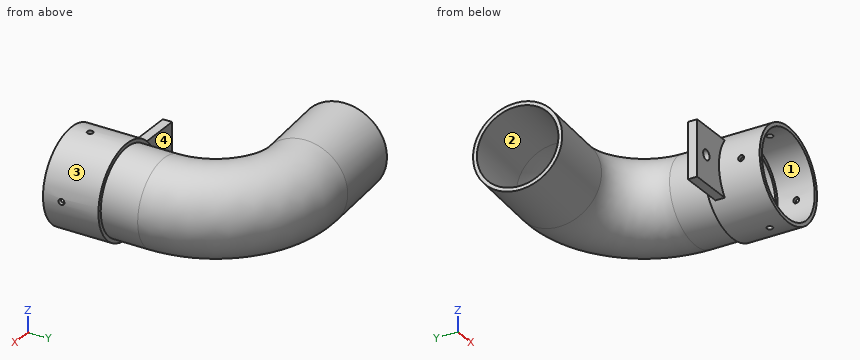
```python
from build123d import *

# Parameters (mm, degrees)
SKETCH_1_R               = 23
SKETCH_1_R_2             = 21
EXTRUDE_1_DEPTH          = 20
EXTRUDE_1_DEPTH_BACK     = 10
SKETCH_3_R               = 25
SKETCH_3_R_2             = 23
SKETCH_5_R               = 2.75
EXTRUDE_3_DEPTH          = 5
CUT_EXTRUDE_1_DEPTH      = 136.900654152
CUT_EXTRUDE_1_DEPTH_BACK = 136.900654152
SKETCH_6_R               = 1.6
CUT_EXTRUDE_2_DEPTH      = 136.900654171
CUT_EXTRUDE_2_DEPTH_BACK = 136.900654171
SKETCH_7_R               = 1.6


with BuildPart() as part:
    # Sweep 1: sweep along a path in Sketch 2
    with BuildLine(Plane.XY) as sweep_1_path:
        Line((0, 0), (0, 30))
        ThreePointArc((0, 30), (-14.598440657, 63.177480156), (-48.922008424, 74.828761414))
        Line((-48.922008424, 74.828761414), (-88.769796347, 71.342531704))
    # Sketch 1 → Sweep 1 (sweep)
    with BuildSketch(Plane(origin=(0, 0, 0), x_dir=(1, 0, 0), z_dir=(0, 1, 0))):
        Circle(SKETCH_1_R)
        Circle(SKETCH_1_R_2, mode=Mode.SUBTRACT)
    sweep(path=sweep_1_path.line)


with BuildPart() as body_2:
    # Sketch 3 → Extrude 1 (new, two sides: drawn at the far end of the back side and taken through both)
    with BuildSketch(Plane(origin=(0, 0, 58.765701135), x_dir=(1, 0, 0), z_dir=(0, -1, 0)).offset(-EXTRUDE_1_DEPTH_BACK)):
        with Locations(Location((0, -58.765701135, 0), (0, 0, 270))):
            Circle(SKETCH_3_R)
        with Locations(Location((0, -58.765701135, 0), (0, 0, 270))):
            Circle(SKETCH_3_R_2, mode=Mode.SUBTRACT)
    extrude(amount=EXTRUDE_1_DEPTH + EXTRUDE_1_DEPTH_BACK)


    add(part.part)  # Extrude 3 merges part
    # Sketch 5 → Extrude 3 (add)
    with BuildSketch(Plane(origin=(0, 2, 0), x_dir=(-1, 0, 0), z_dir=(0, -1, 0))):
        with BuildLine():
            Line((20, 15), (44, 15))
            Line((44, 15), (44, -15))
            Line((44, -15), (20, -15))
            ThreePointArc((20, -15), (25, 0), (20, 15))
        make_face()
        with Locations(Location((36, 0, 0), (0, 0, 90))):
            Circle(SKETCH_5_R, mode=Mode.SUBTRACT)
    extrude(amount=-EXTRUDE_3_DEPTH)

    # Sketch 6 → Cut-Extrude 1 (cut, two sides: drawn at the far end of the back side and taken through both)
    with BuildSketch(Plane(origin=(0, 0, 0), x_dir=(0, 0, -1), z_dir=(1, 0, 0)).offset(-CUT_EXTRUDE_1_DEPTH_BACK)):
        with Locations((0, -10)):
            Circle(SKETCH_6_R)
    extrude(amount=CUT_EXTRUDE_1_DEPTH + CUT_EXTRUDE_1_DEPTH_BACK, mode=Mode.SUBTRACT)

    # Sketch 7 → Cut-Extrude 2 (cut, two sides: drawn at the far end of the back side and taken through both)
    with BuildSketch(Plane.XY.offset(-CUT_EXTRUDE_2_DEPTH_BACK)):
        with Locations((0, -10)):
            Circle(SKETCH_7_R)
    extrude(amount=CUT_EXTRUDE_2_DEPTH + CUT_EXTRUDE_2_DEPTH_BACK, mode=Mode.SUBTRACT)


solid = body_2.part
```
Input: part model. Units: mm. Frame: model coordinates. Face numbers are marked on the shaded views. Round coordinates to 2 decimals unless told otherwise and drop trailing zeros. Loops run counter-clockwise (first coordinate to the right, second up) from the corner with the lowest first, then second, coordinate; pieces in that order, holes last. Notation, with made-up numbers: (82, 40) -> (100, 40) arc R18 cw to (100, 71) -> close; hole circle Ø2 at (-34.75, -37.5). An arc over 180 degrees is marked (long way). Use one line per item in the form item = value. Start each with the question number.
Item 1: Material intervals for L1, parallel to Y at x = 24, z = 0; L2, parallel to Y at x = -36, z = 8; L3, parallel to Y at x = -34, z = -2, sorted ascending. Write a range as from..to.
Item 2: Section query D-D on y = 22. Return the cut outline in (x, z).
Item 3: Section query B-B on y = -10. Return the cut outline in (x, z).
Item 4: Section query C-C on x = 0. Count the separate pieces of the cut face and the enclosed holes in it, then the cut area to 3 significant figures.
Item 5: Mould query, pull axis X, two halves, no side actions, for the marked faces 1, 2, 3 and 4. Classes: pulls with the +X half, pulls with the -X half, needs draft (parallel to the pull), parting line crosses it, or undercut.
Item 6: Section query A-A on z = -6.5. Return the cut outline in (x, y), then the cut area to 3 significant figures.
Item 7: Contact query for flat-ended pins moving along their axis: pin 1 Ø1.5 at (y, z) = (5.5, -5) entering from -X; pin 2 Ø3.5 at (x, z) = (-36, 0) entering from +Y; pin 3 Ø2 at (x, z) = (-51.5, 15) entering from +Y; pin 4 Ø4 at (x, y) = (0, -10) entering from -Z. Output: stop coordinate, or through.
Ans:
q1.L1 = -20..-11.6, -8.4..10
q1.L2 = 2..7, 51.64..53.95, 93.78..95.95
q1.L3 = 2..7, 49.15..51.44, 94.98..97.02
q2.outline = circle Ø46 at (0, 0); hole circle Ø42 at (0, 0)
q3.outline = (-24.95, -1.6) arc R25 ccw to (-1.6, -24.95) -> (-1.6, -22.94) arc R23 cw to (-22.94, -1.6) -> close; (-24.95, 1.6) -> (-22.94, 1.6) arc R23 cw to (-1.6, 22.94) -> (-1.6, 24.95) arc R25 ccw to start; (1.6, -24.95) arc R25 ccw to (24.95, -1.6) -> (22.94, -1.6) arc R23 cw to (1.6, -22.94) -> close; (1.6, 22.94) arc R23 cw to (22.94, 1.6) -> (24.95, 1.6) arc R25 ccw to (1.6, 24.95) -> close
q4.separate_pieces = 3
q4.enclosed_holes = 0
q4.area = 497 mm^2
q5.face_1 = undercut
q5.face_2 = undercut
q5.face_3 = parting line crosses it
q5.face_4 = needs draft
q6.outline = (-90.69, 93.32) -> (-90.51, 91.24) -> (-50.66, 94.72) arc R64.97 cw to (19.97, 30) -> (19.97, 0) -> (22.06, 0) -> (22.06, -20) -> (24.14, -20) -> (24.14, 10) -> (22.06, 10) -> (22.06, 30) arc R67.06 ccw to (-50.84, 96.81) -> close; (-87.03, 51.45) -> (-86.85, 49.36) -> (-47, 52.85) arc R22.94 cw to (-22.06, 30) -> (-22.06, 10) -> (-24.14, 10) -> (-24.14, 7) -> (-44, 7) -> (-44, 2) -> (-24.14, 2) -> (-24.14, -20) -> (-22.06, -20) -> (-22.06, 0) -> (-19.97, 0) -> (-19.97, 30) arc R25.03 ccw to (-47.18, 54.94) -> close
q6.area = 830 mm^2
q7.pin_1 = -44
q7.pin_2 = 97.61
q7.pin_3 = 92.93
q7.pin_4 = -25
